For this review, take the finished solid that the model builds, in its own axes (mm). Face numbers are marked on the shaded views. Give positions to 0.01 mm unless a question says otherwise; leave off trailing zeros. Loops run counter-clockwise (first coordinate to the right, second up) from the corner with the lowest first, then second, coordinate; pieces in that order, holes last.
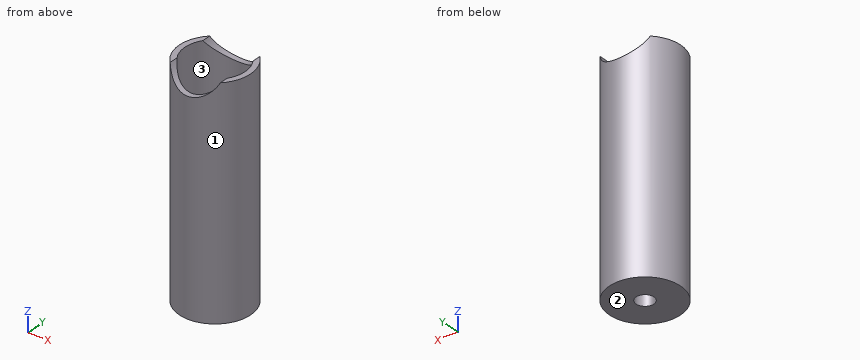
```python
from build123d import *

# Parameters (mm, degrees)
F3_DEPTH      = 12.801
F3_DEPTH_BACK = 12.801


with BuildPart() as f1:
    # F0 (on Front) → F1 (revolve)
    with BuildSketch(Plane.XZ):
        Polygon((3.2, 0), (12.8, 0), (12.8, 80), (10.8, 80), (10.8, 10), (5.2, 10), (4.4, 10.8), (4.4, 12.9607695155), (3.8, 14), (3.2, 14), align=None)
    revolve(axis=Axis((0, 0, 37.0239801705), (0, 0, 1)))

    # F2 (on Front) → F3 (cut, two sides)
    with BuildSketch(Plane.XZ) as f3_sk:
        with BuildLine():
            Line((9, 80), (-9, 80))
            ThreePointArc((-9, 80), (0, 74), (9, 80))
        make_face()
    extrude(amount=-F3_DEPTH, mode=Mode.SUBTRACT)
    extrude(f3_sk.sketch, amount=F3_DEPTH_BACK, mode=Mode.SUBTRACT)


solid = f1.part
```
Item 1: Take a section at C-C on z = 39.5. Give the boundary of the cut face in (x, y), and give its area (3 significant figures).
Answer:
outline: circle Ø25.6 at (0, 0); hole circle Ø21.6 at (0, 0)
area: 148 mm2
Item 2: The part is to be moulded in two halves that separate along Y. For the marked faces 1, 2 and 3, say which applies: released by +Y, released by -Y, zero draft, split by the parting line, or undercut.
Answer:
face 1: split by the parting line
face 2: zero draft
face 3: undercut
Item 3: Take a section at A-A on x = 0. Give the boundary of the cut face in (y, z).
Answer:
outline: (-12.8, 0) - (-3.2, 0) - (-3.2, 14) - (-3.8, 14) - (-4.4, 12.96) - (-4.4, 10.8) - (-5.2, 10) - (-10.8, 10) - (-10.8, 74) - (-12.8, 74) - close; (3.2, 0) - (12.8, 0) - (12.8, 74) - (10.8, 74) - (10.8, 10) - (5.2, 10) - (4.4, 10.8) - (4.4, 12.96) - (3.8, 14) - (3.2, 14) - close
Item 4: Take a section at B-B on y = 0. Give the boundary of the cut face in (x, z).
Answer:
outline: (-12.8, 0) - (-3.2, 0) - (-3.2, 14) - (-3.8, 14) - (-4.4, 12.96) - (-4.4, 10.8) - (-5.2, 10) - (-10.8, 10) - (-10.8, 80) - (-12.8, 80) - close; (3.2, 0) - (12.8, 0) - (12.8, 80) - (10.8, 80) - (10.8, 10) - (5.2, 10) - (4.4, 10.8) - (4.4, 12.96) - (3.8, 14) - (3.2, 14) - close
Item 5: Clearance check with flat-ended pins moving along their axes: pin 1 Ø4 at (x, y) = (0, -1.5) entering from +Z; pin 2 Ø2 at (x, y) = (9, -3) entering from +Z; pin 3 Ø3 at (x, z) = (8.5, 28) entering from -Y. State where each tip first meets the part, or that it passes through.
Answer:
pin 1: stops at z = 14
pin 2: stops at z = 10
pin 3: stops at y = -10.72
Item 6: For L1, parallel to Y at x = 0, z = 9.5; L2, parallel to X at y = 0, z = 57; L3, parallel to Y at x = 0, z = 10.25, list the stretches that pass through material, from the lowest coordinate up.
Answer:
L1: y = -12.8 to -3.2, 3.2 to 12.8
L2: x = -12.8 to -10.8, 10.8 to 12.8
L3: y = -12.8 to -10.8, -4.95 to -3.2, 3.2 to 4.95, 10.8 to 12.8
Item 7: Take a section at D-D on z = 5. Give the boundary of the cut face in (x, y).
Answer:
outline: circle Ø25.6 at (0, 0); hole circle Ø6.4 at (0, 0)
